Verification items for the finished model (mm, model axes). Coordinates: 2 decimals unless noted, no trailing zeros. Write each loop counter-clockwise with the first axis right and the second up, starting at its lowest first coordinate (ties: lowest second). Pieces come first, ordered by that corner, then holes. Notation, with made-up numbers: (57, -14.5) -> (86, -14.5) arc R15 ccw to (86, 2.5) -> close; hole circle Ø1 at (73.25, 76.25). An arc over 180 degrees is marked (long way). Answer in a Markdown table with one row per item.
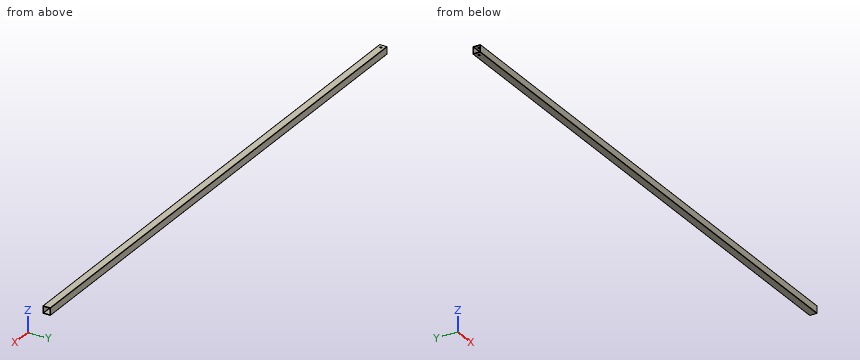
```python
from build123d import *

# Parameters (mm, degrees)
BOSS_EXTRUDE1_DEPTH      = 914.4
BOSS_EXTRUDE1_DEPTH_BACK = 914.4
SKETCH5_R                = 3.81
CUT_EXTRUDE1_DEPTH       = 915.840865943


with BuildPart() as part:
    # Sketch4 → Boss-Extrude1 (new, two sides: drawn at the far end of the back side and taken through both)
    with BuildSketch(Plane(origin=(0, 0, 0), x_dir=(0, 0, -1), z_dir=(1, 0, 0)).offset(-BOSS_EXTRUDE1_DEPTH_BACK)):
        with BuildLine():
            Line((12.7, -11.43), (12.7, 11.43))
            ThreePointArc((12.7, 11.43), (12.328025612, 12.328025612), (11.43, 12.7))
            Line((11.43, 12.7), (-11.43, 12.7))
            ThreePointArc((-11.43, 12.7), (-12.328025612, 12.328025612), (-12.7, 11.43))
            Line((-12.7, 11.43), (-12.7, -11.43))
            ThreePointArc((-12.7, -11.43), (-12.328025612, -12.328025612), (-11.43, -12.7))
            Line((-11.43, -12.7), (11.43, -12.7))
            ThreePointArc((11.43, -12.7), (12.328025612, -12.328025612), (12.7, -11.43))
        make_face()
        with BuildLine():
            Line((10.5918, 9.53262), (10.5918, -9.53262))
            ThreePointArc((10.5918, -9.53262), (10.28157336, -10.28157336), (9.53262, -10.5918))
            Line((9.53262, -10.5918), (-9.53262, -10.5918))
            ThreePointArc((-9.53262, -10.5918), (-10.28157336, -10.28157336), (-10.5918, -9.53262))
            Line((-10.5918, -9.53262), (-10.5918, 9.53262))
            ThreePointArc((-10.5918, 9.53262), (-10.28157336, 10.28157336), (-9.53262, 10.5918))
            Line((-9.53262, 10.5918), (9.53262, 10.5918))
            ThreePointArc((9.53262, 10.5918), (10.28157336, 10.28157336), (10.5918, 9.53262))
        make_face(mode=Mode.SUBTRACT)
    extrude(amount=BOSS_EXTRUDE1_DEPTH + BOSS_EXTRUDE1_DEPTH_BACK)

    # Sketch5 → Cut-Extrude1 (cut, through all)
    with BuildSketch(Plane.XY.offset(12.7)):
        with Locations((-901.7, 0)):
            Circle(SKETCH5_R)
    extrude(amount=-CUT_EXTRUDE1_DEPTH, mode=Mode.SUBTRACT)


solid = part.part
```
1. Sectioned sample at C-C, the plane x = 23.5. Record the cut outline in (y, z).
Findings below:
| item | result |
|---|---|
| outline | (-12.7, -11.43) arc R1.27 ccw to (-11.43, -12.7) -> (11.43, -12.7) arc R1.27 ccw to (12.7, -11.43) -> (12.7, 11.43) arc R1.27 ccw to (11.43, 12.7) -> (-11.43, 12.7) arc R1.27 ccw to (-12.7, 11.43) -> close; hole (-10.59, -9.53) arc R1.06 ccw to (-9.53, -10.59) -> (9.53, -10.59) arc R1.06 ccw to (10.59, -9.53) -> (10.59, 9.53) arc R1.06 ccw to (9.53, 10.59) -> (-9.53, 10.59) arc R1.06 ccw to (-10.59, 9.53) -> close |
2. Material ranges on probe 1 along Z at (x, y) = (-398.5, 7.5); probe 2 along Y at (x, z) = (-901.7, -12), recorded low to high. Write a range as from..to.
Findings below:
| item | result |
|---|---|
| probe 1 | z = -12.7..-10.59, 10.59..12.7 |
| probe 2 | y = -12.56..-3.81, 3.81..12.56 |
3. Sectioned sample at A-A, the plane y = 0. Record the cut outline in (x, z), and give its area (3 significant figures).
Findings below:
| item | result |
|---|---|
| outline | (-914.4, -12.7) -> (-905.51, -12.7) -> (-905.51, -10.59) -> (-914.4, -10.59) -> close; (-914.4, 10.59) -> (-905.51, 10.59) -> (-905.51, 12.7) -> (-914.4, 12.7) -> close; (-897.89, -12.7) -> (914.4, -12.7) -> (914.4, -10.59) -> (-897.89, -10.59) -> close; (-897.89, 10.59) -> (914.4, 10.59) -> (914.4, 12.7) -> (-897.89, 12.7) -> close |
| area | 7,680 mm² |
4. Sectioned sample at B-B, the plane z = 4.25. Record the cut outline in (x, y).
Findings below:
| item | result |
|---|---|
| outline | (-914.4, -12.7) -> (914.4, -12.7) -> (914.4, -10.59) -> (-914.4, -10.59) -> close; (-914.4, 10.59) -> (914.4, 10.59) -> (914.4, 12.7) -> (-914.4, 12.7) -> close |
